Read the model definition and answer for the solid it produces. Units are mm, in the model's axes. Face numbers are marked on the shaded views. A direction names the side the tool comes from. Coordinates: 2 decimals unless noted, no trailing zeros. Order: outer loops, then holes, each group sorted by start corner. A loop starts at its lowest first (then second) coordinate and runs counter-clockwise, first axis right, second up.
from build123d import *

# Parameters (mm, degrees)
SKETCH_1_R      = 3.35
EXTRUDE_1_DEPTH = 100


with BuildPart() as part:
    # 草图1 → 凸台-拉伸1 (new body)
    with BuildSketch(Plane.XY):
        with BuildLine():
            Line((-5.8, -4.244365081), (-9.805634919, -8.25))
            Line((-9.805634919, -8.25), (-12.8, -8.25))
            Line((-12.8, -8.25), (-12.8, -4.1))
            Line((-12.8, -4.1), (-14, -4.1))
            Line((-14, -4.1), (-14, -5.2))
            Line((-14, -5.2), (-15, -5.2))
            Line((-15, -5.2), (-15, -12.5))
            ThreePointArc((-15, -12.5), (-14.267766953, -14.267766953), (-12.5, -15))
            Line((-12.5, -15), (42.5, -15))
            ThreePointArc((42.5, -15), (44.267766953, -14.267766953), (45, -12.5))
            Line((45, -12.5), (45, -5.2))
            Line((45, -5.2), (44, -5.2))
            Line((44, -5.2), (44, -4.1))
            Line((44, -4.1), (42.8, -4.1))
            Line((42.8, -4.1), (42.8, -8.25))
            Line((42.8, -8.25), (39.805634919, -8.25))
            Line((39.805634919, -8.25), (35.8, -4.244365081))
            Line((35.8, -4.244365081), (35.8, 4.244365081))
            Line((35.8, 4.244365081), (39.805634919, 8.25))
            Line((39.805634919, 8.25), (42.8, 8.25))
            Line((42.8, 8.25), (42.8, 4.1))
            Line((42.8, 4.1), (44, 4.1))
            Line((44, 4.1), (44, 5.2))
            Line((44, 5.2), (45, 5.2))
            Line((45, 5.2), (45, 12.5))
            ThreePointArc((45, 12.5), (44.267766953, 14.267766953), (42.5, 15))
            Line((42.5, 15), (35.2, 15))
            Line((35.2, 15), (35.2, 14))
            Line((35.2, 14), (34.1, 14))
            Line((34.1, 14), (34.1, 12.8))
            Line((34.1, 12.8), (38.25, 12.8))
            Line((38.25, 12.8), (38.25, 9.805634919))
            Line((38.25, 9.805634919), (34.244365081, 5.8))
            Line((34.244365081, 5.8), (25.755634919, 5.8))
            Line((25.755634919, 5.8), (21.75, 9.805634919))
            Line((21.75, 9.805634919), (21.75, 12.8))
            Line((21.75, 12.8), (25.9, 12.8))
            Line((25.9, 12.8), (25.9, 14))
            Line((25.9, 14), (24.8, 14))
            Line((24.8, 14), (24.8, 15))
            Line((24.8, 15), (5.2, 15))
            Line((5.2, 15), (5.2, 14))
            Line((5.2, 14), (4.1, 14))
            Line((4.1, 14), (4.1, 12.8))
            Line((4.1, 12.8), (8.25, 12.8))
            Line((8.25, 12.8), (8.25, 9.805634919))
            Line((8.25, 9.805634919), (4.244365081, 5.8))
            Line((4.244365081, 5.8), (-4.244365081, 5.8))
            Line((-4.244365081, 5.8), (-8.25, 9.805634919))
            Line((-8.25, 9.805634919), (-8.25, 12.8))
            Line((-8.25, 12.8), (-4.1, 12.8))
            Line((-4.1, 12.8), (-4.1, 14))
            Line((-4.1, 14), (-5.2, 14))
            Line((-5.2, 14), (-5.2, 15))
            Line((-5.2, 15), (-12.5, 15))
            ThreePointArc((-12.5, 15), (-14.267766953, 14.267766953), (-15, 12.5))
            Line((-15, 12.5), (-15, 5.2))
            Line((-15, 5.2), (-14, 5.2))
            Line((-14, 5.2), (-14, 4.1))
            Line((-14, 4.1), (-12.8, 4.1))
            Line((-12.8, 4.1), (-12.8, 8.25))
            Line((-12.8, 8.25), (-9.805634919, 8.25))
            Line((-9.805634919, 8.25), (-5.8, 4.244365081))
            Line((-5.8, 4.244365081), (-5.8, -4.244365081))
        make_face()
        with Locations((30, 0)):
            Circle(SKETCH_1_R, mode=Mode.SUBTRACT)
        Circle(SKETCH_1_R, mode=Mode.SUBTRACT)
        Polygon((38.25, -9.805634919), (34.244365081, -5.8), (25.755634919, -5.8), (21.75, -9.805634919), (21.75, -12.8), (38.25, -12.8), align=None, mode=Mode.SUBTRACT)
        Polygon((8.25, -9.805634919), (4.244365081, -5.8), (-4.244365081, -5.8), (-8.25, -9.805634919), (-8.25, -12.8), (8.25, -12.8), align=None, mode=Mode.SUBTRACT)
        Polygon((19.55, 12.8), (10.45, 12.8), (10.45, 8.894365081), (5.8, 4.244365081), (5.8, -4.244365081), (10.45, -8.894365081), (10.45, -12.8), (19.55, -12.8), (19.55, -8.894365081), (24.2, -4.244365081), (24.2, 4.244365081), (19.55, 8.894365081), align=None, mode=Mode.SUBTRACT)
    extrude(amount=EXTRUDE_1_DEPTH)


solid = part.part
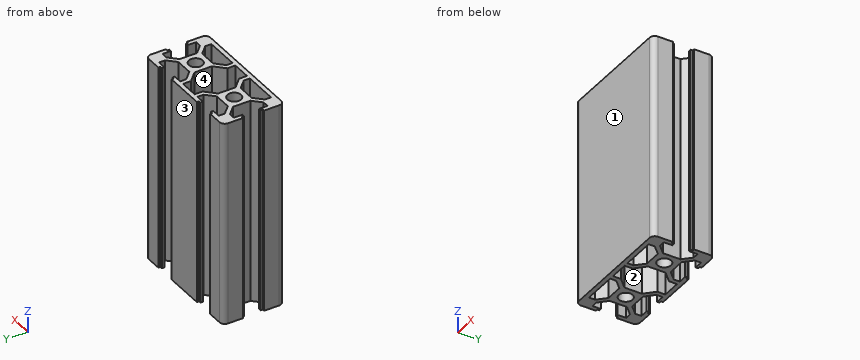
Q1. Which of the six approach directions +Z, -Z, +X, -X, +Y, -Y give full straight-line access (tool end or side, diameter ignored) to the marked faces 1 and 2?
Q2. Each of these flat-tipped pins is pushed along its axis until it touches: P1, Ø4, axis at x = 30, y = 0, coming from the -Z side; P2, Ø0.6, axis at y = -4.5, z = 35, coming from the -X side; P3, Ø1, axis at y = -0.5, z = 26, coming from the -X side. Where does it stop, or does it pass through?
Q3. The part is cut by section D-D, the plane x = -7. Determine the outline of the cut face in (y, z).
Q4. The part is cut by section C-C, the plane y = 0. Determine the outline of the cut face in (x, z), then the cut area to 3 significant figures.
Q5. The part is cut by section B-B, the plane x = 11.5. Determine the outline of the cut face in (y, z), then the cut area to 3 significant figures.
Q6. Determine the mould class of the marked faces 3 and 4 for opening direction X: +X half, -X half, draft (parallel to the pull), parting line (faces both ways), or undercut.
Q7. Straight lines are drawn through the part: L1, parallel to Y at x = 0, z = 35.5; L2, parallel to X at y = -0.25, z = 31.5; L3, parallel to X at y = -4.25, z = 36. For each, find the intervals that lie inside material, in ascending order.
Q8. The part is cut by section A-A, the plane x = 0. Determine the outline of the cut face in (y, z).
Computed values:
1. face 1: +Z, -Z, +X, -X, -Y
1. face 2: +Z, -Z
2. P1: passes through
2. P2: stops at x = -14
2. P3: stops at x = -5.8
3. outline: (-15, 0) - (-12.8, 0) - (-12.8, 100) - (-15, 100) - close; (-8.56, 0) - (-5.44, 0) - (-5.44, 100) - (-8.56, 100) - close; (5.44, 0) - (8.56, 0) - (8.56, 100) - (5.44, 100) - close; (12.8, 0) - (15, 0) - (15, 100) - (12.8, 100) - close
4. outline: (-5.8, 0) - (-3.35, 0) - (-3.35, 100) - (-5.8, 100) - close; (3.35, 0) - (5.8, 0) - (5.8, 100) - (3.35, 100) - close; (24.2, 0) - (26.65, 0) - (26.65, 100) - (24.2, 100) - close; (33.35, 0) - (35.8, 0) - (35.8, 100) - (33.35, 100) - close
4. area: 980 mm2
5. outline: (-15, 0) - (-12.8, 0) - (-12.8, 100) - (-15, 100) - close; (12.8, 0) - (15, 0) - (15, 100) - (12.8, 100) - close
5. area: 440 mm2
6. face 3: draft
6. face 4: undercut
7. L1: y = -15 to -12.8, -5.8 to -3.35, 3.35 to 5.8
7. L2: x = -5.8 to -3.34, 3.34 to 5.8, 24.2 to 26.66, 33.34 to 35.8
7. L3: x = -14 to -12.8, -5.81 to 5.81, 24.19 to 35.81, 42.8 to 44
8. outline: (-15, 0) - (-12.8, 0) - (-12.8, 100) - (-15, 100) - close; (-5.8, 0) - (-3.35, 0) - (-3.35, 100) - (-5.8, 100) - close; (3.35, 0) - (5.8, 0) - (5.8, 100) - (3.35, 100) - close
